Can you work these out from the drawing? Everything is in mm from the part's minimum corner. A direction names the side the tool comes from. Give positions to 0.01 mm unless a question says otherwise; leave off trailing zeros. Write each loop counter-clockwise with the first axis right and the second up, starting at its lowest first coordinate (ties: lowest second). Pieces come first, ordered by that corner, then holes. Notation, with made-up numbers: (8, 86) -> (24, 86) arc R17 ccw to (24, 104) -> close; hole circle Ø3 at (-12, 32). An arc over 180 degrees is marked (long way). Answer as CSV lines item,"result". Start each with the question number.
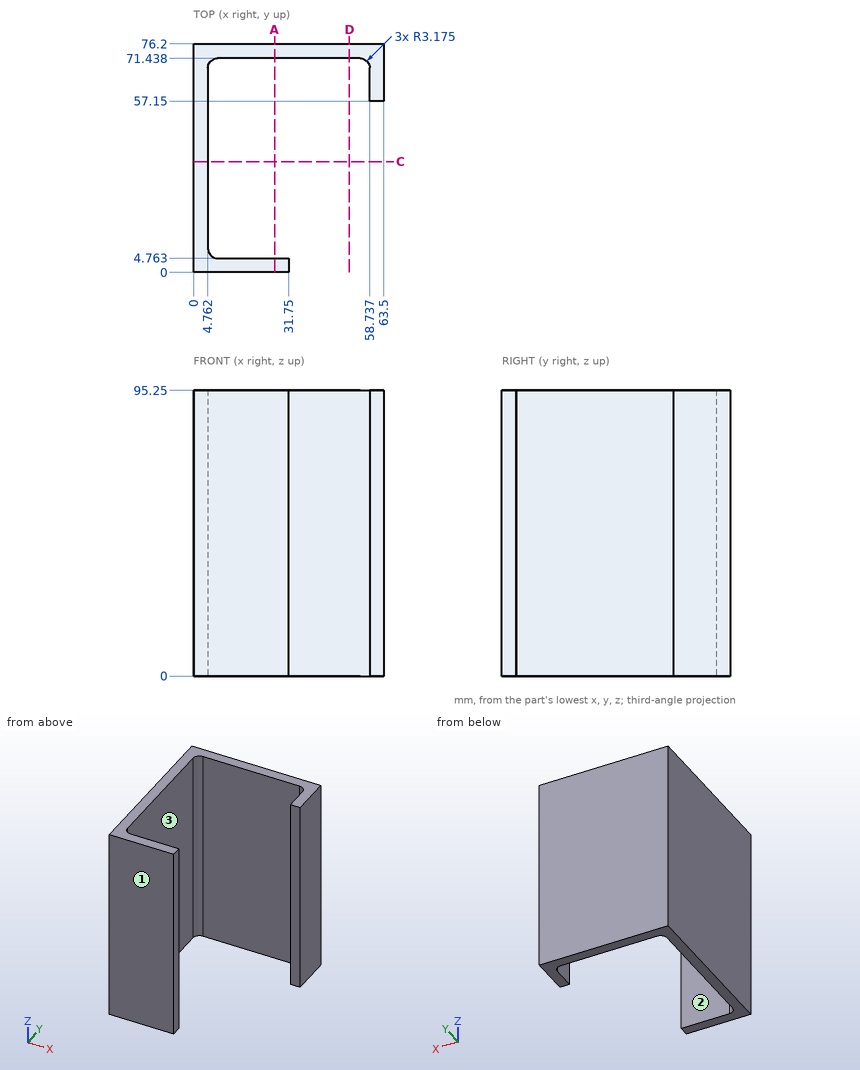
Item 1: If we section it at A-A (x = 27): Please give me the cut outline in (y, z).
Item 2: If we section it at D-D (x = 52): Please give me the cut outline in (y, z).
Item 3: If we section it at C-C (y = 37): Please give me the cut outline in (x, z).
Item 4: I'm going to push flat-ended pins straight in: pin 1 (2 mm diameter, centred on x = 9, y = 68.5, fed in from +Z); pin 2 (12 mm diameter, centred on y = 15.5, z = 20.5, fed in from +X); pin 3 (1.4 mm diameter, centred on y = 2.5, z = 24, fed in from +X); pin 4 (2 mm diameter, centred on x = 45, z = 78, fed in from -Y). Where does each tip first touch, or does it pass through?
Item 5: If I drill on line 1 (Y direction, x = 23, z = 53); line 2 (X direction, y = 67, z = 76); line 3 (Y direction, x = 44, z = 91), over which ranges is the centre line in solid material (lowest first)? Write a range as [from, to].
Item 6: For the marked faces 1, 2 and 3, which set-ups out of +Z, -Z, +X, -X, +Y, -Y let a thin tool reach every point of the face, with its end or its side?
Final values:
1,outline,"(0, 0) -> (4.76, 0) -> (4.76, 95.25) -> (0, 95.25) -> close; (71.44, 0) -> (76.2, 0) -> (76.2, 95.25) -> (71.44, 95.25) -> close"
2,outline,"(71.44, 0) -> (76.2, 0) -> (76.2, 95.25) -> (71.44, 95.25) -> close"
3,outline,"(0, 0) -> (4.76, 0) -> (4.76, 95.25) -> (0, 95.25) -> close"
4,pin 1,"through"
4,pin 2,"x = 4.76"
4,pin 3,"x = 31.75"
4,pin 4,"y = 71.44"
5,line 1,"[0, 4.76], [71.44, 76.2]"
5,line 2,"[0, 4.76], [58.74, 63.5]"
5,line 3,"[71.44, 76.2]"
6,face 1,"+Z, -Z, +X, -X, -Y"
6,face 2,"+Z, -Z, +X"
6,face 3,"+Z, -Z"
